CAD build for the part. Positions are in the model's coordinates, mm. Coordinates: 2 decimals unless noted, no trailing zeros. Loops run counter-clockwise (first coordinate to the right, second up) from the corner with the lowest first, then second, coordinate; pieces in that order, holes last. Notation, with made-up numbers: (-25.5, 64.5) - (27.5, 64.5) arc R10 cw to (27.5, 70.5) - close; hole circle Ø3 at (-31.75, -32). An arc over 180 degrees is marked (long way). Put each result on its own line as item: value.
```python
from build123d import *

# Parameters (mm, degrees)
F0_W     = 76.2
F0_H     = 76.2
F1_DEPTH = 3.175
F2_SIZE  = 50.8
F3_R     = 5.08
F5_D     = 6.35


with BuildPart() as f1:
    # F0 (on Front) → F1 (new body)
    with BuildSketch(Plane.XZ):
        with Locations((38.1, 38.1)):
            Rectangle(F0_W, F0_H)
    extrude(amount=F1_DEPTH)

    # F2
    f2_edges = [f1.edges().sort_by_distance(p)[0] for p in [
        (76.2, -1.5875, 76.2),
    ]]
    chamfer(f2_edges, length=F2_SIZE)

    # F3
    f3_edges = [f1.edges().sort_by_distance(p)[0] for p in [
        (0, -1.5875, 76.2),
        (25.4, -1.5875, 76.2),
        (76.2, -1.5875, 25.4),
        (76.2, -1.5875, 0),
        (0, -1.5875, 0),
    ]]
    fillet(f3_edges, radius=F3_R)

    # F5 (through all)
    with Locations(Plane(origin=(0, 0, 0), x_dir=(-1, 0, 0), z_dir=(0, 1, 0))):
        with Locations((-12.7, 12.7), (-12.7, 38.1), (-12.7, 63.5), (-38.1, 12.7), (-63.5, 12.7)):
            Hole(F5_D / 2)


solid = f1.part
```
Q1. Mould opens along X. For faces 1 (the flat face through (29, 0, 30)), 2 (the cylindrical face through (25.27, -1.61, 75.8)), 3 (the cylindrical face through (10.36, -1.61, 65.646)) say: +X half, -X half, draft (parallel to the pull), parting line (faces both ways), or undercut.
Determined:
face 1: draft
face 2: +X half
face 3: undercut
Q2. Slice it at C-C, the plane z = 38.1. Give the cut face in (x, y) (3 decimals).
Determined:
outline: (0, -3.175) - (9.525, -3.175) - (9.525, 0) - (0, 0) - close; (15.875, -3.175) - (63.5, -3.175) - (63.5, 0) - (15.875, 0) - close
Q3. Slice it at B-B, the plane z = 12.7. Give the cut face in (x, y) (3 decimals), then the cut area to 3 significant figures.
Determined:
outline: (0, -3.175) - (9.525, -3.175) - (9.525, 0) - (0, 0) - close; (15.875, -3.175) - (34.925, -3.175) - (34.925, 0) - (15.875, 0) - close; (41.275, -3.175) - (60.325, -3.175) - (60.325, 0) - (41.275, 0) - close; (66.675, -3.175) - (76.2, -3.175) - (76.2, 0) - (66.675, 0) - close
area: 181 mm2
Q4. Slice it at D-D, the plane y = -2.3. Give the cut face in (x, z) (3 decimals).
Determined:
outline: (0, 5.08) arc R5.08 ccw to (5.08, 0) - (71.12, 0) arc R5.08 ccw to (76.2, 5.08) - (76.2, 23.296) arc R5.08 ccw to (74.712, 26.888) - (26.888, 74.712) arc R5.08 ccw to (23.296, 76.2) - (5.08, 76.2) arc R5.08 ccw to (0, 71.12) - close; hole circle Ø6.35 at (12.7, 12.7); hole circle Ø6.35 at (12.7, 38.1); hole circle Ø6.35 at (12.7, 63.5); hole circle Ø6.35 at (38.1, 12.7); hole circle Ø6.35 at (63.5, 12.7)
Q5. Wall check: L1, parallel to Z at x = 12.7, y = -1.7 (3 decimals); L2, parallel to X at y = -0.7, z = 15; L3, parallel to X at y = -1.5, z = 13.5. Give the ranges that are in metal, low to high. Write a range as from..to.
Determined:
L1: 0..9.525, 15.875..34.925, 41.275..60.325, 66.675..76.2
L2: 0..10.51, 14.89..35.91, 40.29..61.31, 65.69..76.2
L3: 0..9.63, 15.77..35.03, 41.17..60.43, 66.57..76.2
Q6. Slice it at A-A, the plane x = 38.1. Give the cut face in (y, z) (3 decimals), then the cut area to 3 significant figures.
Determined:
outline: (-3.175, 0) - (0, 0) - (0, 9.525) - (-3.175, 9.525) - close; (-3.175, 15.875) - (0, 15.875) - (0, 63.5) - (-3.175, 63.5) - close
area: 181 mm2
